Work out the finished part from the listing and answer in its coordinate system (mm). A direction names the side the tool comes from. Coordinates: 2 decimals unless noted, no trailing zeros. Loops run counter-clockwise (first coordinate to the right, second up) from the corner with the lowest first, then second, coordinate; pieces in that order, holes last. Notation, with made-up numbers: (38.5, 16.5) -> (46.5, 16.5) arc R14 ccw to (46.5, 35.5) -> close; hole circle Ø7 at (57, 31). An arc over 180 degrees is marked (long way). Use a Markdown table: item, result.
Autodesk Inventor part; units mm, degrees
ref_plane "РабПлоскость3" through (2, 0, 0) normal (1, 0, 0) x (0, 1, 0)
ref_plane "XZ Plane" through (0, 0, 0) normal (0, 1, 0) x (-1, 0, 0)
ref_plane "XY Plane" through (0, 0, 0) normal (0, 0, 1) x (1, 0, 0)
sketch "Эскиз1" plane through (0, 0, 0) normal (1, 0, 0) x (0, 1, 0)
  circle A0 centre (0, 0) radius 33
  circle A1 centre (0, 0) radius 27.5
  line L0 (27.5, 0) -> (12.5, 0)
  line L1 (0, 27.5) -> (0, 12.5)
  arc A2 (0, -12.5) -> (12.5, 0) centre (0, 0) ccw
  arc A3 (-12.5, 0) -> (0, -12.5) centre (0, 0) ccw
  arc A4 (0, 12.5) -> (-12.5, 0) centre (0, 0) ccw
  arc A5 (12.5, 0) -> (0, 12.5) centre (0, 0) ccw
  line L2 (27.5, 0) -> (22.5, 0)
  line L3 (0, -27.5) -> (0, -22.5)
  line L4 (27.5, 0) -> (22.5, 0)
  line L5 (0, 27.5) -> (0, 22.5)
  line L6 (-27.5, 0) -> (-22.5, 0)
  circle A6 centre (0, 0) radius 22.5
  line L7 (-8.8388, -8.8388) -> (-15.9436, -15.8761)
  line L8 (-12.5, 0) -> (-22.5, 0)
  line L9 (-8.8388, 8.8388) -> (-15.8761, 15.9436)
  line L10 (8.8388, 8.8388) -> (16.0277, 15.7912)
  line L11 (12.5, 0) -> (22.5, 0)
  line L12 (0, 12.5) -> (0, 22.5)
  line L13 (8.8388, -8.8388) -> (15.7912, -16.0277)
  line L14 (0, -22.5) -> (0, -12.5)
  circle A7 centre (0, 0) radius 27.5
  circle A8 centre (0, 0) radius 32
  point P0 (-27.5, 0)
  point P1 (0, 22.5)
  point P2 (0, 22.5)
  point P3 (-22.5, 0)
  point P4 (-22.5, 0)
  dimension "d2" = 15
  dimension "d3" = 15
  dimension "d4" = 15
  dimension "d5" = 15
  dimension "d21" = 5
  dimension "d22" = 5
  dimension "d25" = 360
  dimension "d67" = 64
extrude "Выдавливание1" add sketch "Эскиз1" along normal blind 15 contours L0 A6 L1 A1 | A1 L3 A6 L0 | L1 A6 L6 A1 | A1 L6 A6 L3 | A6 L13 A2 L0 | L0 A5 L10 A6 | A6 L10 A5 L1 | L1 A4 L9 A6 | L14 A2 L13 A6 | A6 L7 A3 L14 | A2 A3 A4 A5 | L8 A3 L7 A6 | A6 L9 A4 L8 | A8
sketch "Эскиз5" plane through (15, 0, 0) normal (1, 0, 0) x (0, 0, -1)
  point P0 (0, 0)
extrude "Выдавливание3" cut sketch "Эскиз1" along normal blind 15 contours L0 A5 L10 A6 | L1 A4 L9 A6 | L14 A2 L13 A6 | L8 A3 L7 A6
sketch "Эскиз6" plane through (15, 0, 0) normal (1, 0, 0) x (0, 0, -1)
  circle A0 centre (0, 0) radius 11.25
  arc A1 (0, 12.5) -> (-8.8388, 8.8388) centre (0, 0) ccw
  arc A2 (0, 12.5) -> (-8.8388, 8.8388) centre (0, 0) ccw
  line L0 (0, 0) -> (-3.0615, 7.391) construction
  circle A3 centre (-3.0615, 7.391) radius 1.5
  circle A4 centre (-7.391, -3.0615) radius 1.5
  circle A5 centre (3.0615, -7.391) radius 1.5
  circle A6 centre (7.391, 3.0615) radius 1.5
  arc A7 (-3.0615, 7.391) -> (-7.391, -3.0615) centre (0, 0) ccw
  line L1 (-8.8388, 8.8388) -> (-22.3952, 22.8573) construction
  circle A8 centre (0, 0) radius 32 construction
  line L2 (-8.8388, 8.8388) -> (10.6622, 8.8388) construction
  arc A9 (-22.3952, 22.8573) -> (-32, 0) centre (0, 0) ccw construction
  line L3 (-29.5012, 12.3966) -> (-7.391, 3.0615)
  dimension "d31" = 22.5
  dimension "d72" = 8
  dimension "d74" = 3
  dimension "d77" = 360
  dimension "d79" = 134.04
extrude "Выдавливание4" [suppressed]
extrude "Выдавливание5" cut sketch "Эскиз6" against normal blind 12 contours A0 | A3 | A4 | A5 | A6
extrude "Выдавливание6" [suppressed]
chamfer "Фаска2" distance 2 angle 45 1 edges at (0, -12.3912, -12.3575)
chamfer "Фаска3" distance 2 angle 45 15 edges at (0, -20.7964, -8.5883) (0, -17.5, 0) (0, -11.5485, -4.7835) (0, 0, -17.5) (0, 8.5331, -20.8191) (0, 12.315, -12.4333) (0, 4.7835, -11.5485) (0, 17.5, 0) (0, 11.5485, 4.7835) (0, 20.8191, 8.5331) (0, 12.4333, 12.315) (0, 0, 17.5) (0, -4.7835, 11.5485) (0, -12.3575, 12.3912) (0, -8.5883, 20.7964)
ref_plane "РабПлоскость3" through (2, 0, 0) normal (1, 0, 0) x (0, 1, 0)
sketch "Эскиз10" plane through (2, 0, 0) normal (1, 0, 0) x (0, 1, 0)
  circle A0 centre (0, 0) radius 26.5
  circle A1 centre (0, 0) radius 27.5
  circle A2 centre (0, 0) radius 26.5
  dimension "d66" = 53
sketch "Эскиз11" plane through (0, 0, 0) normal (-1, 0, 0) x (0, 0, 1)
  circle A0 centre (0, 0) radius 31
  circle A1 centre (0, 0) radius 32
  dimension "d68" = 62
extrude "Выдавливание9" cut sketch "Эскиз11" against normal blind 11 from surface at -2
extrude "Выдавливание10" cut sketch "Эскиз6" against normal blind 15 contours A3 | A5
chamfer "Фаска4" distance 2 angle 45 2 edges at (0, 7.391, 4.5615) (0, -7.391, -1.5615)
sketch "Эскиз12" plane through (15, 0, 0) normal (1, 0, 0) x (0, 0, -1)
  circle A0 centre (0, 0) radius 32
  arc A1 (0, 12.5) -> (-8.8388, 8.8388) centre (0, 0) ccw
  line L0 (-8.8388, 8.8388) -> (-22.3952, 22.8573)
  circle A2 centre (0, 0) radius 32
  line L1 (-8.8388, 8.8388) -> (10.6622, 8.8388) construction
  point P0 (0, 0)
  point P1 (-32, 0)
  dimension "d85" = 134.04
ref_plane "РабПлоскость4" through (15, 12.3966, 29.5012) normal (0, 0.387395, 0.9219138) x (-1, 0, 0)
sketch "Эскиз14" plane through (15, 12.3966, 29.5012) normal (0, 0.387395, 0.9219138) x (-1, 0, 0)
  circle A0 centre (8, 0) radius 2.25
  point P0 (15, 0)
  dimension "d87" = 4.5
extrude "Выдавливание11" cut sketch "Эскиз14" against normal blind 25
sketch "Эскиз15" plane through (3, 0, 0) normal (1, 0, 0) x (0, 0, -1)
  circle A0 centre (0, 0) radius 2
  dimension "d90" = 4
properties part number "колеса прототип"
Q1. Given pin 1 Ø8 at (y, z) = (5, 6.5) entering from +X; pin 2 Ø3.5 at (y, z) = (7.39, 3.06) entering from +X; pin 3 Ø8 at (x, z) = (7.5, 17.5) entering from -Y; pin 4 Ø3 at (x, y) = (10, -16.5) entering from -Z, each flat-ended and moving along its own axis, determine where each tip first touches the part or whether it passes through.
Solved:
| item | result |
|---|---|
| pin 1 | x = 15 |
| pin 2 | x = 3 |
| pin 3 | y = -27.91 |
| pin 4 | z = -27.13 |
Q2. For faces 1 (the flat face through (2, 29, -12)), 2 (the flat face through (1.01, -12.89, 11.52)), 3 (the flat face through (8, 18, 0)), determine the directions among +Z, -Z, +X, -X, +Y, -Y from which every point of the face is accessible in a straight line to the end or side of a thin tool.
Solved:
| item | result |
|---|---|
| face 1 | none |
| face 2 | -X |
| face 3 | +X, -X |
Q3. Determine the mould class of faces 4 (the cylindrical face through (13.99, -6.94, 31.24)), 5 (the flat face through (13, 29, -12)), 6 (the cylindrical face through (8.41, -20.75, -8.7)) for opening direction Z: pulls with the +Z half, pulls with the -Z half, needs draft (parallel to the pull), parting line crosses it, or undercut.
Solved:
| item | result |
|---|---|
| face 4 | parting line crosses it |
| face 5 | needs draft |
| face 6 | undercut |
Q4. Section B-B on x = 6 is taken. Determine the outline of the cut face in (y, z), and give its area (3 significant figures).
Solved:
| item | result |
|---|---|
| outline | (2.43, 10.98) -> (10.13, 29.3) arc R31 ccw (long way) to (13.84, 27.74) -> (6.15, 9.42) arc R11.25 cw (long way) to start; hole (-22.5, 0) arc R22.5 ccw to (-15.94, -15.88) -> (-8.84, -8.84) arc R12.5 cw to (-12.5, 0) -> close; hole (-15.88, 15.94) -> (-8.84, 8.84) arc R12.5 cw to (0, 12.5) -> (0, 22.5) arc R22.5 ccw to start; hole (0, -22.5) arc R22.5 ccw to (15.79, -16.03) -> (8.84, -8.84) arc R12.5 cw to (0, -12.5) -> close; hole (8.84, 8.84) arc R12.5 cw to (12.5, 0) -> (22.5, 0) arc R22.5 ccw to (16.03, 15.79) -> close |
| area | 1,990 mm² |
Q5. Section A-A on x = 11.75 is taken. Determine the outline of the cut face in (y, z), and give its area (3 significant figures).
Solved:
| item | result |
|---|---|
| outline | circle Ø62 at (0, 0); hole (-22.5, 0) arc R22.5 ccw to (-15.94, -15.88) -> (-8.84, -8.84) arc R12.5 cw to (-12.5, 0) -> close; hole (-15.88, 15.94) -> (-8.84, 8.84) arc R12.5 cw to (0, 12.5) -> (0, 22.5) arc R22.5 ccw to start; hole circle Ø22.5 at (0, 0); hole (0, -22.5) arc R22.5 ccw to (15.79, -16.03) -> (8.84, -8.84) arc R12.5 cw to (0, -12.5) -> close; hole (8.84, 8.84) arc R12.5 cw to (12.5, 0) -> (22.5, 0) arc R22.5 ccw to (16.03, 15.79) -> close |
| area | 2,070 mm² |
Q6. Section C-C on y = -15 is taken. State how many separate pieces and enclosed holes the cut face has, and give its area (3 significant figures).
Solved:
| item | result |
|---|---|
| separate pieces | 3 |
| enclosed holes | 0 |
| area | 563 mm² |
Q7. Consider line 1 (Y direction, x = 9, z = -6.5); line 2 (Y direction, x = 13.5, z = -6); line 3 (Z direction, x = 0.5, y = 8). Determine where each line is inside the solid, lowest interval first. Write a range as [from, to].
Solved:
| item | result |
|---|---|
| line 1 | [-30.31, -21.54], [-10.68, -9.18], [9.18, 30.31] |
| line 2 | [-31.43, -21.69], [-10.97, -9.52], [9.52, 31.43] |
| line 3 | [-30.98, -22.63], [-7.55, 0.12], [6, 7.55], [10.11, 30.98] |
